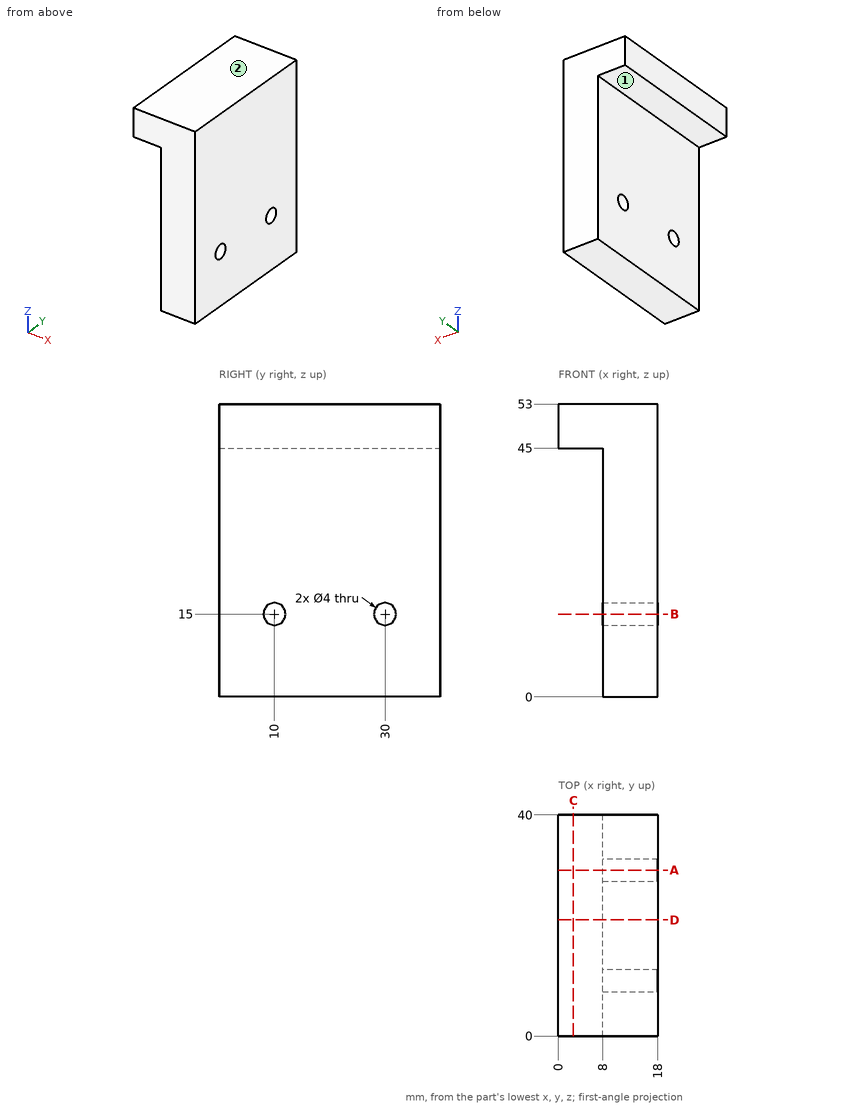
Study the drawing (mm; zero at the part's minimum x, y, z) and answer. A direction names the side the tool comes from. Round coordinates to 2 decimals unless told otherwise and drop trailing zeros. Write each loop counter-clockwise with the first axis right and the second up, starting at its lowest first coordinate (ties: lowest second). Pieces come first, ordered by that corner, then holes.
Q1. Find section B-B on z = 15. Determine the outline of the cut face in (x, y).
Values:
outline: (8, 0) - (18, 0) - (18, 8) - (8, 8) - close; (8, 12) - (18, 12) - (18, 28) - (8, 28) - close; (8, 32) - (18, 32) - (18, 40) - (8, 40) - close
Q2. A tool of negligible diameter and unlimited length cuts with its end or side. For the marked faces 1 and 2, from which of +Z, -Z, +X, -X, +Y, -Y can it reach the whole face along a straight path? Write none if from no direction.
Values:
face 1: -Z, -X, +Y, -Y
face 2: +Z, +X, -X, +Y, -Y
Q3. Find section D-D on y = 21. Determine the outline of the cut face in (x, z).
Values:
outline: (0, 45) - (8, 45) - (8, 0) - (18, 0) - (18, 53) - (0, 53) - close
Q4. Straight lines are drawn through the part: line 1 (Z direction, x = 14, y = 10); line 2 (Z direction, x = 7.75, y = 17); line 3 (Z direction, x = 10, y = 9.5). For each, find the intervals that lie inside material, in ascending order.
Values:
line 1: z = 0 to 13, 17 to 53
line 2: z = 45 to 53
line 3: z = 0 to 13.06, 16.94 to 53
Q5. Flat-ended cylindrical pins translate along their axes: P1, Ø5, axis at y = 30, z = 15, coming from the -X side; P2, Ø2.5, axis at y = 10, z = 15, coming from the +X side; P3, Ø4, axis at x = 4.5, y = 14.5, coming from the -Z side. Find the tip coordinate at first contact, or state that the pin passes through.
Values:
P1: stops at x = 8
P2: passes through
P3: stops at z = 45
Q6. Find section A-A on y = 30. Determine the outline of the cut face in (x, z), and give its area (3 significant figures).
Values:
outline: (0, 45) - (8, 45) - (8, 17) - (18, 17) - (18, 53) - (0, 53) - close; (8, 0) - (18, 0) - (18, 13) - (8, 13) - close
area: 554 mm2
Q7. Find section C-C on x = 2.75. Determine the outline of the cut face in (y, z).
Values:
outline: (0, 45) - (40, 45) - (40, 53) - (0, 53) - close
